Could you check a few things on this model? Use its own coordinates, in mm. Face numbers are marked on the shaded views. A direction names the side the tool comes from. Coordinates: 2 decimals unless noted, no trailing zeros. Order: outer loops, then holes, each group sorted by start corner. A loop starts at its lowest first (then second) coordinate and runs counter-clockwise, first axis right, second up. Notation, with made-up numbers: (78.5, 86) - (118.5, 86) arc R21 cw to (118.5, 121) - close; hole circle Ø6 at (24.5, 50.5). An arc over 180 degrees is marked (long way). Answer as a JSON object with one key per item and string values. Group by question number.
(1) Imagine slicing it at D-D, the plane z = 5. Write out the boundary of the cut face in (x, y).
(2) Which directions (+Z, -Z, +X, -X, +Y, -Y) give clear straight access to the entire face, cutting with the end or side of a thin tool? Please do the marked faces 1 and 2.
(3) Imagine slicing it at B-B, the plane y = 5. Write out the boundary of the cut face in (x, z), and give its area (3 significant figures).
(4) Imagine slicing it at C-C, the plane x = -0.5. Write out the boundary of the cut face in (y, z), and give its area (3 significant figures).
(5) We'd pull the mould along X, two halves only. Please class the marked faces 3, 4 and 5: pulls with the +X half, pulls with the -X half, needs draft (parallel to the pull), parting line crosses it, or undercut.
(6) Imagine slicing it at A-A, the plane x = 19. Write out the boundary of the cut face in (y, z), and give its area (3 significant figures).
(7) Please list where these lines run through material, in increasing order: probe 1 along Y at (x, z) = (14.5, 5); probe 2 along X at (y, z) = (-18, 7.25); probe 3 along Z at (x, y) = (17.5, -36.2).
(8) Will this pin go through, and if not, where does the flat tip stop? P1, Ø1.5, axis at x = 18, z = 4.5, coming from the -Y side.
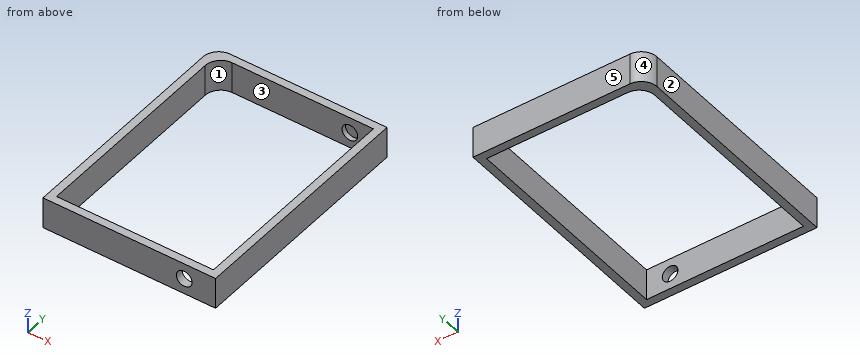
from build123d import *

# Parameters (mm, degrees)
SKETCH_1_W          = 55
SKETCH_1_H          = 75
EXTRUDE_1_DEPTH     = 10
SKETCH_3_W          = 50
SKETCH_3_H          = 70
CUT_EXTRUDE_1_DEPTH = 48.565743976
FILLET_2_R          = 5
SKETCH_4_R          = 2.5
CUT_EXTRUDE_2_DEPTH = 1.5
SKETCH_5_R          = 2.5
CUT_EXTRUDE_3_DEPTH = 79.182478856


with BuildPart() as part:
    # 草图1 → 凸台-拉伸1 (new body)
    with BuildSketch(Plane.XY):
        Rectangle(SKETCH_1_W, SKETCH_1_H)
    extrude(amount=EXTRUDE_1_DEPTH)

    # 草图3 → 切除-拉伸1 (cut, through all)
    with BuildSketch(Plane(origin=(0, 0, 0), x_dir=(-1, 0, 0), z_dir=(0, 0, -1))):
        Rectangle(SKETCH_3_W, SKETCH_3_H)
    extrude(amount=-CUT_EXTRUDE_1_DEPTH, mode=Mode.SUBTRACT)

    # 圆角2
    fillet_2_edges = [part.edges().sort_by_distance(p)[0] for p in [
        (-25, 35, 5),
        (-27.5, 37.5, 5),
    ]]
    fillet(fillet_2_edges, radius=FILLET_2_R)

    # 草图4 → 切除-拉伸2 (cut)
    with BuildSketch(Plane.XZ.offset(-35)):
        with Locations((17.5, 5)):
            Circle(SKETCH_4_R)
    extrude(amount=-CUT_EXTRUDE_2_DEPTH, mode=Mode.SUBTRACT)

    # 草图5 → 切除-拉伸3 (cut, through all)
    with BuildSketch(Plane(origin=(0, -35, 0), x_dir=(1, 0, 0), z_dir=(0, 1, 0))):
        with Locations((17.5, -5)):
            Circle(SKETCH_5_R)
    extrude(amount=-CUT_EXTRUDE_3_DEPTH, mode=Mode.SUBTRACT)


solid = part.part
Result set:
{
 "1": {"outline": "(-27.5, -37.5) - (15, -37.5) - (15, -35) - (-25, -35) - (-25, 30) arc R5 cw to (-20, 35) - (15, 35) - (15, 36.5) - (20, 36.5) - (20, 35) - (25, 35) - (25, -35) - (20, -35) - (20, -37.5) - (27.5, -37.5) - (27.5, 37.5) - (-22.5, 37.5) arc R5 ccw to (-27.5, 32.5) - close"},
 "2": {"face 1": "+Z, -Z", "face 2": "+Z, -Z, -X, +Y, -Y"},
 "3": {"outline": "(-27.5, 0) - (-25, 0) - (-25, 10) - (-27.5, 10) - close; (25, 0) - (27.5, 0) - (27.5, 10) - (25, 10) - close", "area": "50.0 mm^2"},
 "4": {"outline": "(-37.5, 0) - (-35, 0) - (-35, 10) - (-37.5, 10) - close; (35, 0) - (37.5, 0) - (37.5, 10) - (35, 10) - close", "area": "50.0 mm^2"},
 "5": {"face 3": "undercut", "face 4": "pulls with the -X half", "face 5": "needs draft"},
 "6": {"outline": "(-37.5, 0) - (-35, 0) - (-35, 3) - (-37.5, 3) - close; (-37.5, 7) - (-35, 7) - (-35, 10) - (-37.5, 10) - close; (35, 0) - (37.5, 0) - (37.5, 10) - (35, 10) - (35, 7) - (36.5, 7) - (36.5, 3) - (35, 3) - close", "area": "34.0 mm^2"},
 "7": {"probe 1": "y = -37.5 to -35, 35 to 37.5", "probe 2": "x = -27.5 to -25, 25 to 27.5", "probe 3": "z = 0 to 2.5, 7.5 to 10"},
 "8": {"P1": "stops at y = 36.5"}
}
